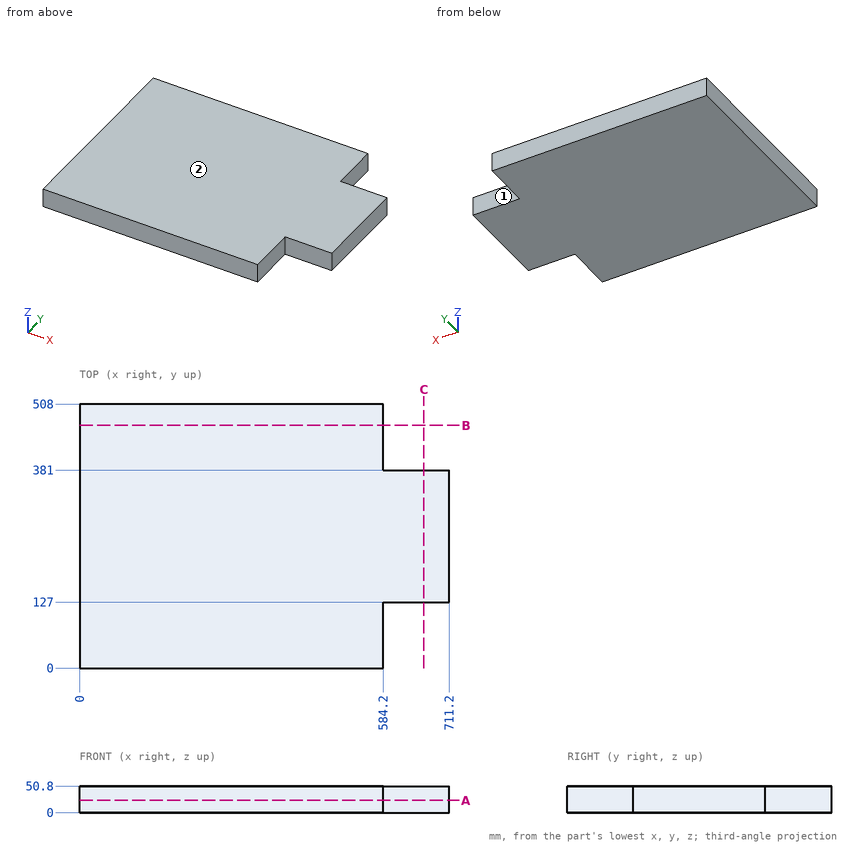
Design review of the part shown in the three views and the two pictorial views. Dimensions are in mm from the part's minimum x, y and z. A direction names the side the tool comes from. Coordinates: 2 decimals unless noted, no trailing zeros. Order: outer loops, then holes, each group sorted by start corner. A loop starts at its lowest first (then second) coordinate and runs counter-clockwise, first axis right, second up. Notation, with made-up numbers: (-36, 31) -> (19, 31) arc R35 cw to (19, 68) -> close; hole circle Ø4 at (47.25, 21). An arc over 180 degrees is marked (long way). Use one line per item in the form item = value. Start each with the question number.
(1) For the marked faces 1 and 2, list the 3-axis set-ups (+Z, -Z, +X, -X, +Y, -Y) from which the entire face can be reached by the end or side of a thin tool; tool diameter is ignored.
(2) Add section B-B on y = 467. State the section outline as (x, z) points, plus the area to 3 significant figures.
(3) Add section A-A on z = 23.5. State the section outline as (x, y) points.
(4) For probe 1 along X at (y, z) = (402.5, 29); probe 2 along Y at (x, z) = (668.5, 21), list the stretches that pass through material, from the lowest coordinate up.
(5) Insertion check: pin 1 (15 mm diameter, centred on y = 462.5, z = 24, fed in from +X). The pin has a flat end and moves straight along its axis. Give the tip position at first contact, or say it passes through.
(6) Add section C-C on x = 662. State the section outline as (y, z) points, plus the area to 3 significant figures.
Answer block:
q1.face_1 = +Z, -Z, +X, +Y
q1.face_2 = +Z, +X, -X, +Y, -Y
q2.outline = (0, 0) -> (584.2, 0) -> (584.2, 50.8) -> (0, 50.8) -> close
q2.area = 29,700 mm²
q3.outline = (0, 0) -> (584.2, 0) -> (584.2, 127) -> (711.2, 127) -> (711.2, 381) -> (584.2, 381) -> (584.2, 508) -> (0, 508) -> close
q4.probe_1 = 0 to 584.2
q4.probe_2 = 127 to 381
q5.pin_1 = 584.2
q6.outline = (127, 0) -> (381, 0) -> (381, 50.8) -> (127, 50.8) -> close
q6.area = 12,900 mm²
